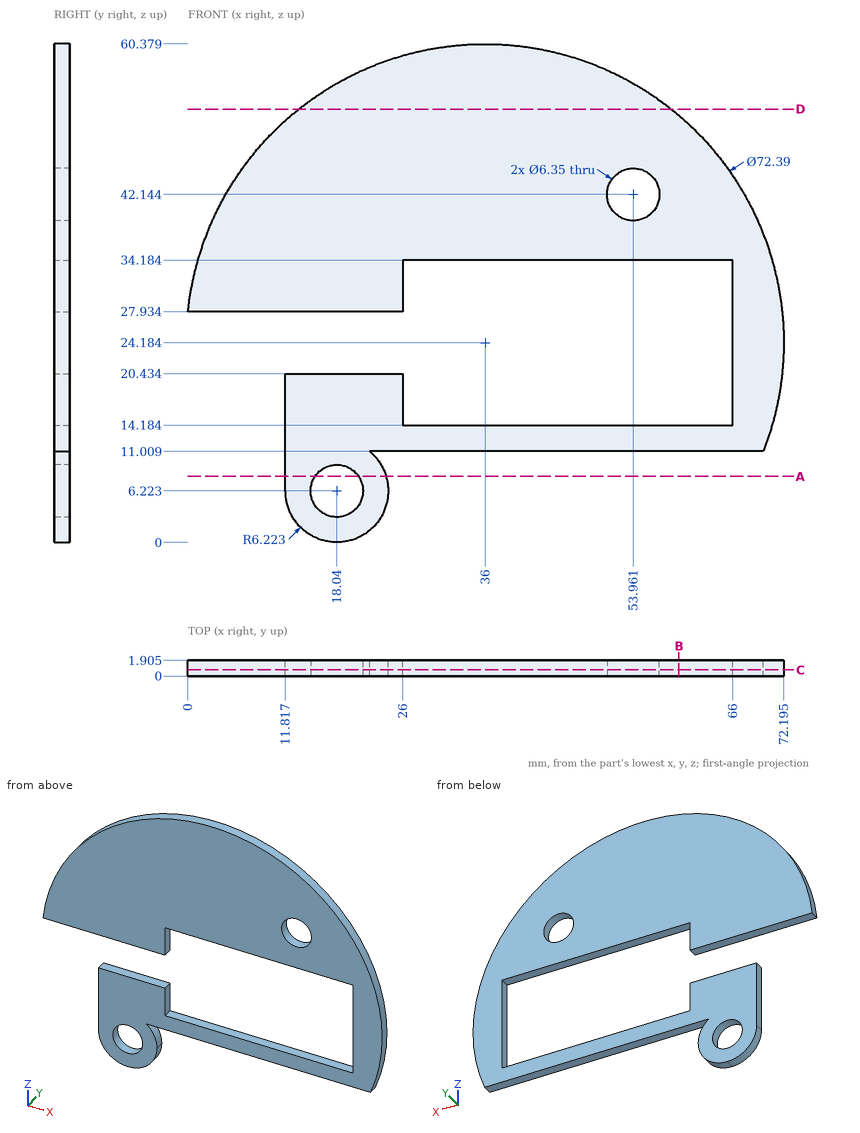
Input: dimensioned drawing with shaded views. Units: mm. Origin: part minimum x, y, z. Coordinates: 2 decimals unless noted, no trailing zeros. Loops run counter-clockwise (first coordinate to the right, second up) from the corner with the lowest first, then second, coordinate; pieces in that order, holes last. Notation, with made-up numbers: M 69,0.5 L 110,0.5 A36 ccw 110,39.5 Z; hole C 76,-14.5 d3. An arc over 180 degrees is marked long. One line per item, written item: value.
(1) Section B-B (x = 59.5). Output: boundary loops of the cut face in (y, z) (1 decimal).
Filled in:
outline: M 0,11 L 1.9,11 L 1.9,14.2 L 0,14.2 Z; M 0,34.2 L 1.9,34.2 L 1.9,51.7 L 0,51.7 Z
(2) Pin query (flat end, axial travel): pin 1 (1 mm diameter, centred on x = 55.5, z = 44.5, fed in from -Y); pin 2 (1 mm diameter, centred on x = 26, y = 0.5, fed in from +Z); pin 3 (1 mm diameter, centred on x = 46.5, y = 0.5, fed in from -Z); pin 4 (1 mm diameter, centred on y = 1, z = 32, fed in from +X). Return the tip coordinate at first contact, or that it passes through.
Filled in:
pin 1: y = 0
pin 2: z = 59.11
pin 3: z = 11.01
pin 4: x = 71.45
(3) Section C-C (y = 0.75). Give the number of separate pieces and of enclosed holes in the cut face.
Filled in:
separate pieces: 1
enclosed holes: 2
(4) Section D-D (z = 52.5). Output: boundary loops of the cut face in (x, y) (1 decimal).
Filled in:
outline: M 13.5,0 L 58.5,0 L 58.5,1.9 L 13.5,1.9 Z
(5) Section A-A (z = 8). Output: boundary loops of the cut face in (x, y) (1 decimal), and give its area (3 significant figures).
Filled in:
outline: M 11.8,0 L 15.4,0 L 15.4,1.9 L 11.8,1.9 Z; M 20.7,0 L 24,0 L 24,1.9 L 20.7,1.9 Z
area: 13.2 mm^2
(6) Line query: line 1 along Z through (x, y) = (15.5, 1) (1 decimal); line 2 along X through (y, z) = (0.7, 14.5) (1 decimal); line 3 along X through (y, z) = (1.1, 8) (1 decimal). Output: solid intervals per line, ascending. Write a range as from..to.
Filled in:
line 1: 0.5..4.3, 8.1..20.4, 27.9..54
line 2: 11.8..26, 66..70.9
line 3: 11.8..15.4, 20.7..24
